The listing builds one solid part. Answer for the finished solid, in the listing's coordinates (mm). A direction names the side the tool comes from. Round coordinates to 2 decimals unless told otherwise and drop trailing zeros. Loops run counter-clockwise (first coordinate to the right, second up) from the corner with the lowest first, then second, coordinate; pieces in that order, holes last. Notation, with made-up numbers: M 5.25,0.5 L 46.25,0.5 A24 cw 46.25,29.5 Z; hole C -20,34 d7. An arc over 180 degrees is marked long. Answer as a JSON object with one key per item and string values.
```python
from build123d import *

# Parameters (mm, degrees)
F0_W           = 25.4
F0_H           = 25.4
F1_DEPTH       = 5.08
F3_D           = 2.3
F3_CSINK_D     = 5
F3_CSINK_ANGLE = 90
F5_DEPTH       = 3.175
F6_R           = 2.2225
F7_DEPTH       = 5.081


with BuildPart() as f1:
    # F0 (on Front) → F1 (new body)
    with BuildSketch(Plane.XZ):
        Rectangle(F0_W, F0_H)
    extrude(amount=F1_DEPTH)

    # F3 (through all)
    with Locations(Plane(origin=(0, 0, 0), x_dir=(1, 0, 0), z_dir=(0, 1, 0))):
        with Locations((6.1722, -7.5438), (-6.1722, 7.5438)):
            CounterSinkHole(F3_D / 2, F3_CSINK_D / 2, counter_sink_angle=F3_CSINK_ANGLE)

    # F4 (on face) → F5 (cut)
    with BuildSketch(Plane.XZ.offset(5.08)):
        Polygon((3.7394976935, 0), (1.8697488468, 3.2385), (-1.8697488468, 3.2385), (-3.7394976935, 0), (-1.8697488468, -3.2385), (1.8697488468, -3.2385), align=None)
    extrude(amount=-F5_DEPTH, mode=Mode.SUBTRACT)

    # F6 (on face) → F7 (cut, through all)
    with BuildSketch(Plane.XZ.offset(5.08)):
        Circle(F6_R)
    extrude(amount=-F7_DEPTH, mode=Mode.SUBTRACT)


solid = f1.part
```
Item 1: The part is cut by section C-C (y = -0.6). Give the vertices of the cut face in (x, z) (1 decimal), then the cut area to 3 significant figures.
Values follow:
{"outline": "M -12.7,-12.7 L 12.7,-12.7 L 12.7,12.7 L -12.7,12.7 Z; hole C -6.2,-7.5 d3.8; hole C 0,0 d4.4; hole C 6.2,7.5 d3.8", "area": "607 mm^2"}
Item 2: Flat-ended cylindrical pins translate along their axes: P1, Ø3.5, axis at x = 6.17, z = 7.54, coming from the +Y side; P2, Ø1.9, axis at x = -1.5, z = -0.5, coming from the -Y side (3 decimals); P3, Ø3.5, axis at x = -6.17, z = -7.54, coming from the -Y side. Find the tip coordinate at first contact, or state that the pin passes through.
Values follow:
{"P1": "y = -0.75", "P2": "y = -1.905", "P3": "y = -5.08"}
Item 3: The part is cut by section B-B (y = -3.95). Give the vertices of the cut face in (x, z), then the cut area to 3 significant figures.
Values follow:
{"outline": "M -12.7,-12.7 L 12.7,-12.7 L 12.7,12.7 L -12.7,12.7 Z; hole C -6.17,-7.54 d2.3; hole M -3.74,0 L -1.87,-3.24 L 1.87,-3.24 L 3.74,0 L 1.87,3.24 L -1.87,3.24 Z; hole C 6.17,7.54 d2.3", "area": "601 mm^2"}
Item 4: The part is cut by section A-A (x = 0). Give the vertices of the cut face in (y, z) (1 decimal).
Values follow:
{"outline": "M -5.1,-12.7 L 0,-12.7 L 0,-2.2 L -1.9,-2.2 L -1.9,-3.2 L -5.1,-3.2 Z; M -5.1,3.2 L -1.9,3.2 L -1.9,2.2 L 0,2.2 L 0,12.7 L -5.1,12.7 Z"}
Item 5: Which of the six approach directions +Z, -Z, +X, -X, +Y, -Y give full straight-line access (tool end or side, diameter ignored) to faces 1 (the face through (2.818, -3.515, 1.597)), 2 (the face through (-0.48, -0.97, -2.17))?
Values follow:
{"face 1": "-Y", "face 2": "+Y, -Y"}
Item 6: Straight lines are drawn through the part: line 1 (Z direction, x = 0, y = -0.9); line 2 (Z direction, x = -6.25, y = -1.65); line 3 (X direction, y = -3, z = -8). For each, find the intervals that lie inside material, in ascending order.
Values follow:
{"line 1": "-12.7 to -2.22, 2.22 to 12.7", "line 2": "-12.7 to -8.69, -6.4 to 12.7", "line 3": "-12.7 to -7.23, -5.12 to 12.7"}
Item 7: Determine the mould class of faces 3 (the face through (-5.92, -3.24, -6.42)), 4 (the face through (3, -5.08, 3)), 5 (the face through (5.11, -3.24, 7.98)), 6 (the face through (-12.7, -3, 0)) for opening direction X: released by +X, released by -X, zero draft, split by the parting line, or undercut.
Values follow:
{"face 3": "undercut", "face 4": "zero draft", "face 5": "undercut", "face 6": "released by -X"}
